```python
from build123d import *

# Parameters (mm, degrees)
SKETCH1_R           = 3
SKETCH1_R_2         = 1.55
BOSS_EXTRUDE1_DEPTH = 14.5
BOSS_EXTRUDE2_START = 14.5
SKETCH1_3_R         = 1.55
BOSS_EXTRUDE2_DEPTH = 2
FILLET1_R           = 0.5


with BuildPart() as part:
    # Sketch1 → Boss-Extrude1 (new body)
    # profile 1 of 2: a face of its own
    with BuildSketch(Plane.XY):
        with Locations(Location((0, 0, 0), (0, 0, 180))):
            Circle(SKETCH1_R)
        Circle(SKETCH1_R_2, mode=Mode.SUBTRACT)
    # profile 2 of 2: a face of its own
    with BuildSketch(Plane.XY):
        Circle(SKETCH1_R_2)
    extrude(amount=BOSS_EXTRUDE1_DEPTH)

    # Sketch1<3> → Boss-Extrude2 (add)
    with BuildSketch(Plane.XY.offset(BOSS_EXTRUDE2_START)):
        Circle(SKETCH1_3_R)
    extrude(amount=BOSS_EXTRUDE2_DEPTH)

    # Fillet1
    fillet1_edges = [part.edges().sort_by_distance(p)[0] for p in [
        (-1.55, 0, 14.5),
    ]]
    fillet(fillet1_edges, radius=FILLET1_R)


solid = part.part
```
CAD build for the part. Positions are in the model's coordinates, mm. A direction names the side the tool comes from. Round coordinates to 2 decimals unless told otherwise and drop trailing zeros. Order: outer loops, then holes, each group sorted by start corner. A loop starts at its lowest first (then second) coordinate and runs counter-clockwise, first axis right, second up. Notation, with made-up numbers: (-11.5, 7.25) - (-4.5, 7.25) arc R26 ccw to (-4.5, 23.25) - close; hole circle Ø7 at (75.25, 18.25). An arc over 180 degrees is marked (long way). Use CSV: the item, a comma, the result in double quotes. Start each with the question number.
1) Saw through at C-C (z = 12.5). List the corners of the cut face in (x, y).
2) Saw through at D-D (x = 2.4). List the corners of the cut face in (y, z).
3) Saw through at A-A (x = 0). List the corners of the cut face in (y, z).
4) Pin check, flat tip, straight feed: pin 1 Ø1 at (x, z) = (1.5, 5) entering from +Y. Stop position of the tip, or through.
5) Tool access for faces 1 (the flat face through (-1, 2, 14.5)), 2 (the cylindrical face through (-2.86, -0.9, 7.15)): list every direction of +Z, -Z, +X, -X, +Y, -Y with a clear straight run to the whole face (end or side of a thin tool).
6) Wall check: L1, parallel to X at y = 0.1, z = 12; L2, parallel to Z at x = -1.15, y = -2. Give the ranges that are in metal, low to high. Write a range as [from, to].
Values follow:
1,outline,"circle Ø6 at (0, 0)"
2,outline,"(-1.8, 0) - (1.8, 0) - (1.8, 14.5) - (-1.8, 14.5) - close"
3,outline,"(-3, 0) - (3, 0) - (3, 14.5) - (2.05, 14.5) arc R0.5 cw to (1.55, 15) - (1.55, 16.5) - (-1.55, 16.5) - (-1.55, 15) arc R0.5 cw to (-2.05, 14.5) - (-3, 14.5) - close"
4,pin 1,"stops at y = 2.83"
5,face 1,"+Z"
5,face 2,"+Z, -Z"
6,L1,"x = [-3, 3]"
6,L2,"z = [0, 14.5]"
